Model file for the job. Use its own axes, mm. Face numbers are marked on the shaded views. A direction names the side the tool comes from. Coordinates: 2 decimals unless noted, no trailing zeros. Order: outer loops, then holes, each group sorted by start corner. A loop starts at its lowest first (then second) coordinate and runs counter-clockwise, first axis right, second up.
from build123d import *

# Parameters (mm, degrees)
SKETCH_2_OUTSIDE_W  = 27.946
SKETCH_2_OUTSIDE_H  = 27.946
CUT_EXTRUDE_1_DEPTH = 10
CHAMFER_1_SIZE      = 1


with BuildPart() as part:
    # Эскиз1 → Повернуть1 (revolve)
    with BuildSketch(Plane.XY, mode=Mode.PRIVATE) as revolve_1_sk:
        Polygon((0, 0), (23, 0), (23, 6), (0, 6), (0, 9), (-6.460769515, 9), (-7.5, 7.2), (-7.5, 0), align=None)
    revolve(revolve_1_sk.sketch.rotate(Axis((0, 0, 0), (1, 0, 0)), 90), axis=Axis((0, 0, 0), (1, 0, 0)))

    # Эскиз2 outside → Вырез-Вытянуть1 (cut)
    with BuildSketch(Plane(origin=(0, 0, 0), x_dir=(0, 0, -1), z_dir=(1, 0, 0))):
        Rectangle(SKETCH_2_OUTSIDE_W, SKETCH_2_OUTSIDE_H)
        Polygon((7.794228634, 4.5), (0, 9), (-7.794228634, 4.5), (-7.794228634, -4.5), (0, -9), (7.794228634, -4.5), align=None, mode=Mode.SUBTRACT)
    extrude(amount=-CUT_EXTRUDE_1_DEPTH, mode=Mode.SUBTRACT)

    # Фаска1
    chamfer_1_edges = [part.edges().sort_by_distance(p)[0] for p in [
        (23, 0, -6),
    ]]
    chamfer(chamfer_1_edges, length=CHAMFER_1_SIZE)


solid = part.part
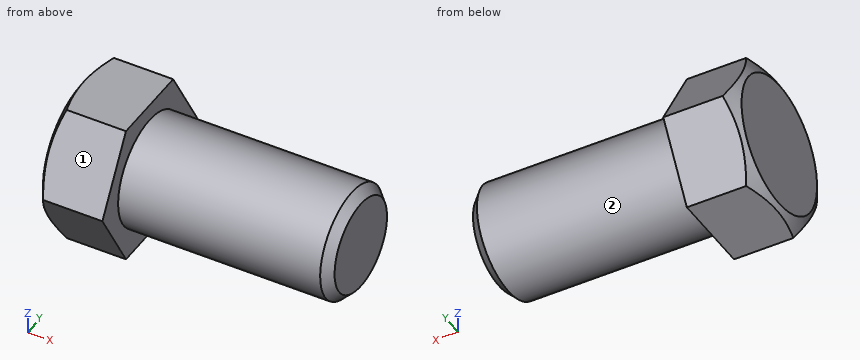
Q1. Cut at B-B, the plane x = 21.5. List the corners of the cut face in (y, z).
Established:
outline: circle Ø12 at (0, 0)
Q2. Cut at A-A, the plane y = 0. List the corners of the cut face in (x, z), plus the area to 3 significant figures.
Established:
outline: (-7.5, -7.2) - (-7.16, -7.79) - (0, -7.79) - (0, -6) - (22, -6) - (23, -5) - (23, 5) - (22, 6) - (0, 6) - (0, 7.79) - (-7.16, 7.79) - (-7.5, 7.2) - close
area: 392 mm2
Q3. Which spindle directions (+Z, -Z, +X, -X, +Y, -Y) get a long thin tool onto all of the face, cutting with end or side? Do the marked faces 1 and 2. Say none if no direction does.
Established:
face 1: +Z, +X, -X, -Y
face 2: +X
Q4. Drop flat-ended pins along their axis: P1, Ø8, axis at x = 6, z = -4, coming from the -Y side; P2, Ø6, axis at x = -1, z = 3.5, coming from the -Y side; P3, Ø1, axis at x = 8, y = 3, coming from the +Z side. Give the stop position or say it passes through.
Established:
P1: stops at y = -6
P2: stops at y = -8.71
P3: stops at z = 5.45
Q5. Probe line 1 (Y direction, x = 14, z = 0.25); line 2 (X direction, y = -0.25, z = -6.75); line 3 (X direction, y = -7.25, z = -1.5). List the from-to ranges inside material, lowest first.
Established:
line 1: y = -5.99 to 5.99
line 2: x = -7.5 to 0
line 3: x = -7.38 to 0
